Source: CAD feature listing. Evaluate the final solid. Frame: model axes, mm. A direction names the side the tool comes from. Give positions to 0.01 mm unless a question says otherwise; leave off trailing zeros. Loops run counter-clockwise (first coordinate to the right, second up) from the corner with the lowest first, then second, coordinate; pieces in that order, holes last.
```python
from build123d import *

# Parameters (mm, degrees)
SKETCH2_R         = 3.207274827
HEX_DIE_DEPTH     = 4.3
FLANGEHEXFILLET_R = 0.2
SKETCH4_R         = 2.40625
INDENT_DEPTH      = 0.358333333


with BuildPart() as part:
    # BodySke → Base-Revolve (revolve)
    with BuildSketch(Plane.XY, mode=Mode.PRIVATE) as base_revolve_sk:
        Polygon((4.3, 2), (4.3, 3.17551963), (0.245673873, 3.17551963), (0, 2.75), (0, 0), (44.3, 0), (44.3, 2), align=None)
    revolve(base_revolve_sk.sketch.rotate(Axis((-25.4, 0, 0), (1, 0, 0)), 90), axis=Axis((-25.4, 0, 0), (1, 0, 0)))

    # Sketch2 → Hex-Die (cut)
    with BuildSketch(Plane(origin=(0, 0, 0), x_dir=(0, 0, -1), z_dir=(1, 0, 0))):
        Circle(SKETCH2_R)
        Polygon((-2.75, 1.587713247), (0, 3.175426494), (2.75, 1.587713247), (2.75, -1.587713247), (0, -3.175426494), (-2.75, -1.587713247), align=None, mode=Mode.SUBTRACT)
    extrude(amount=HEX_DIE_DEPTH, mode=Mode.SUBTRACT)

    # Sketch5 → Flange (revolve)
    with BuildSketch(Plane.XY, mode=Mode.PRIVATE) as flange_sk:
        with BuildLine():
            Line((2.243064243, 0), (3.718092214, 4.052606043))
            ThreePointArc((3.718092214, 4.052606043), (4.052094453, 4.245442326), (4.3, 3.95))
            Line((4.3, 3.95), (4.3, 0))
            Line((4.3, 0), (2.243064243, 0))
        make_face()
    revolve(flange_sk.sketch.rotate(Axis((0, 0, 0), (1, 0, 0)), 90), axis=Axis((0, 0, 0), (1, 0, 0)))

    # FlangeHexFillet
    flangehexfillet_edges = [part.edges().sort_by_distance(p)[0] for p in [
        (3.285203168, 0.797319684, 2.75),
        (3.24398239, 2.381569871, 1.375),
        (3.24398239, 2.381569871, -1.375),
        (3.243982387, 0, -2.75),
        (3.24398239, -2.381569871, -1.375),
        (3.24398239, -2.381569871, 1.375),
        (3.285203168, -0.797319684, 2.75),
    ]]
    fillet(flangehexfillet_edges, radius=FLANGEHEXFILLET_R)

    # Sketch4 → Indent (cut)
    with BuildSketch(Plane(origin=(0, 0, 0), x_dir=(0, 0, -1), z_dir=(1, 0, 0))):
        with Locations(Location((0, 0, 0), (0, 0, 180))):
            Circle(SKETCH4_R)
    extrude(amount=INDENT_DEPTH, mode=Mode.SUBTRACT)


solid = part.part
```
(1) Mould query, pull axis Z, two halves, no side actions, for faces 1 (the flat face through (44.3, 0, 0)), 2 (the flat face through (2, 0, 2.75)), 3 (the conical face through (0.09, -1.46, -2.51)), 4 (the flat face through (0.358, 0, 0)). Classes: pulls with the +Z half, pulls with the -Z half, needs draft (parallel to the pull), parting line crosses it, or undercut.
A:
face 1: needs draft
face 2: pulls with the +Z half
face 3: pulls with the -Z half
face 4: undercut
(2) First-contact query: pin 1 (2 mm diameter, centred on y = 1.5, z = -3, fed in from +X); pin 2 (3 mm diameter, centred on y = -0.5, z = 3, fed in from +X); pin 3 (1 mm diameter, centred on x = 2, y = -0.5, fed in from -Z); pin 4 (4 mm diameter, centred on x = 20, y = -2, fed in from +Z). Flat tips, straight axial feed; report the tip coordinate or a pass-through.
A:
pin 1: stops at x = 4.3
pin 2: stops at x = 44.3
pin 3: stops at z = -2.75
pin 4: stops at z = 2
(3) Ray query, line 1 along Y through (x, z) = (0.3, 0); line 2 along X through (y, z) = (-0.75, 1.75); line 3 along X through (y, z) = (-1, 2.25). Return the intervals inside material, ascending.
A:
line 1: y = -3.18 to -2.41, 2.41 to 3.18
line 2: x = 0.36 to 44.3
line 3: x = 0 to 4.3
(4) Reachability of faces 5 (the cylindrical face through (24, 2, 0)), 6 (the flat face through (1.602, 2.37, 1.394)), 7 (the cylindrical face through (0.177, 1.464, -1.91)) from +Z, -Z, +X, -X, +Y, -Y: full face, straight path, thin tool, end or side. Return the list, or none.
A:
face 5: +X
face 6: +Z, -X, +Y
face 7: -X
(5) Section A-A, the plane x = 6. Return the cut outline in (y, z), then the cut area to 3 significant figures.
A:
outline: circle Ø4 at (0, 0)
area: 12.6 mm2
